```python
from build123d import *

# Parameters (mm, degrees)
SKETCH_1_W                  = 69.5
SKETCH_1_H                  = 55
HOLE_WIZARD_1_D             = 135
HOLE_WIZARD_1_DEPTH         = 13
SKETCH_4_R                  = 15
EXTRUDE_1_DEPTH             = 8
HOLE_WIZARD_M22_1_D         = 26
HOLE_WIZARD_M22_1_DEPTH     = 8
EXTRUDE_2_DEPTH             = 5
CUT_EXTRUDE_START           = -5
CUT_EXTRUDE_1_DEPTH         = 5
CUT_EXTRUDE_2_DEPTH         = 5
CUT_EXTRUDE_3_DEPTH         = 5
HOLE_WIZARD_2_D             = 135
HOLE_WIZARD_2_DEPTH         = 40
THICKEN_START               = -4.2
THICKEN_1_OUTLINE_W         = 3
THICKEN_1_OUTLINE_H         = 6
THICKEN_1_DEPTH             = 8.4
SKETCH_13_W                 = 5
SKETCH_13_H                 = 5
SKETCH_14_W                 = 5
SKETCH_14_H                 = 5
SKETCH_15_W                 = 5
SKETCH_15_H                 = 5
SKETCH_16_W                 = 5
SKETCH_16_H                 = 5
SKETCH_17_W                 = 5
SKETCH_17_H                 = 5
SKETCH_18_W                 = 5
SKETCH_18_H                 = 5
SKETCH_19_W                 = 2.5
SKETCH_19_H                 = 37
SKETCH_20_W                 = 2.5
SKETCH_20_H                 = 37
SKETCH_21_W                 = 2.5
SKETCH_21_H                 = 37
SKETCH_22_W                 = 2.5
SKETCH_22_H                 = 37
HOLE_WIZARD_6_5_6_5_1_D     = 6.5
HOLE_WIZARD_6_5_6_5_1_DEPTH = 3.4
HOLE_WIZARD_15_0_15_1_D     = 15
HOLE_WIZARD_15_0_15_1_DEPTH = 15
HOLE_WIZARD_6_0_6_1_D       = 6
HOLE_WIZARD_6_0_6_1_DEPTH   = 29.048717705
RIB_START                   = -1
RIB_1_OUTLINE_W             = 1
RIB_1_OUTLINE_H             = 4
RIB_1_DEPTH                 = 2
RIB_2_OUTLINE_W             = 4
RIB_2_OUTLINE_H             = 1
RIB_2_DEPTH                 = 2
RIB_3_OUTLINE_W             = 4
RIB_3_OUTLINE_H             = 1
RIB_3_DEPTH                 = 2
RIB_4_OUTLINE_W             = 4
RIB_4_OUTLINE_H             = 1
RIB_4_DEPTH                 = 2


# Read off the part's stored shape, not the designer's step: 切除-加厚1, 筋1, 筋2, 筋3, 筋4
with BuildPart() as part:
    # 草图1 → 旋转1 (revolve)
    with BuildSketch(Plane.XZ, mode=Mode.PRIVATE) as revolve_1_sk:
        with Locations((34.75, 27.5)):
            Rectangle(SKETCH_1_W, SKETCH_1_H)
    revolve(revolve_1_sk.sketch.rotate(Axis((0, 0, 55), (0, 0, -1)), 180), axis=Axis((0, 0, 55), (0, 0, -1)))

    # 孔1
    with Locations(Plane.XY.offset(55)):
        with Locations((0, 0)):
            Hole(HOLE_WIZARD_1_D / 2, depth=HOLE_WIZARD_1_DEPTH)

    # 草图4 → 凸台-拉伸1 (add)
    with BuildSketch(Plane.XY.offset(42)):
        with Locations(Location((0, 0, 0), (0, 0, 180))):
            Circle(SKETCH_4_R)
    extrude(amount=EXTRUDE_1_DEPTH)

    # M22 间隙孔1
    with Locations(Plane.XY.offset(50)):
        with Locations((0, 0)):
            Hole(HOLE_WIZARD_M22_1_D / 2, depth=HOLE_WIZARD_M22_1_DEPTH)

    # 草图7 → 凸台-拉伸2 (add)
    with BuildSketch(Plane.XY.offset(42)):
        with BuildLine():
            Line((12.961481397, -1), (1, -1))
            Line((1, -1), (1, -12.961481397))
            ThreePointArc((1, -12.961481397), (-9.192388155, 9.192388155), (12.961481397, -1))
        make_face()
    extrude(amount=EXTRUDE_2_DEPTH)

    # 草图8 → 切除-拉伸1 (cut)
    with BuildSketch(Plane.XY.offset(47).offset(CUT_EXTRUDE_START)):
        with BuildLine():
            Line((-1, -12.961481397), (-1, -1))
            Line((-1, -1), (-12.961481397, -1))
            ThreePointArc((-12.961481397, -1), (-9.192388155, -9.192388155), (-1, -12.961481397))
        make_face()
    extrude(amount=CUT_EXTRUDE_1_DEPTH, mode=Mode.SUBTRACT)

    # 草图9 → 切除-拉伸2 (cut)
    with BuildSketch(Plane.XY.offset(47).offset(CUT_EXTRUDE_START)):
        with BuildLine():
            Line((-12.961481397, 1), (-1, 1))
            Line((-1, 1), (-1, 12.961481397))
            ThreePointArc((-1, 12.961481397), (-9.192388155, 9.192388155), (-12.961481397, 1))
        make_face()
    extrude(amount=CUT_EXTRUDE_2_DEPTH, mode=Mode.SUBTRACT)

    # 草图10 → 切除-拉伸3 (cut)
    with BuildSketch(Plane.XY.offset(47).offset(CUT_EXTRUDE_START)):
        with BuildLine():
            Line((1, 12.961481397), (1, 1))
            Line((1, 1), (12.961481397, 1))
            ThreePointArc((12.961481397, 1), (9.192388155, 9.192388155), (1, 12.961481397))
        make_face()
    extrude(amount=CUT_EXTRUDE_3_DEPTH, mode=Mode.SUBTRACT)

    # 孔2
    with Locations(Plane(origin=(0, 0, 0), x_dir=(-1, 0, 0), z_dir=(0, 0, -1))):
        with Locations((0, 0)):
            Hole(HOLE_WIZARD_2_D / 2, depth=HOLE_WIZARD_2_DEPTH)

    # 切除-加厚1 outline → 切除-加厚1 (cut)
    with BuildSketch(Plane(origin=(0, 0, 0), x_dir=(0.5591929034707426, 0.8290375725550445, 0), z_dir=(0.8290375725550445, -0.5591929034707428, 0)).offset(THICKEN_START)):
        with Locations((-68.5, 3)):
            Rectangle(THICKEN_1_OUTLINE_W, THICKEN_1_OUTLINE_H)
    extrude(amount=THICKEN_1_DEPTH, mode=Mode.SUBTRACT)

    # 草图13 → 旋转2 (revolve)
    with BuildSketch(Plane.XZ.offset(25), mode=Mode.PRIVATE) as revolve_2_sk:
        with Locations((45.801270189, 44.5)):
            Rectangle(SKETCH_13_W, SKETCH_13_H)
    revolve(revolve_2_sk.sketch.rotate(Axis((43.301270189, -25, 47), (0, 0, -1)), 180), axis=Axis((43.301270189, -25, 47), (0, 0, -1)))

    # 草图14 → 旋转3 (revolve)
    with BuildSketch(Plane.XZ.offset(-25), mode=Mode.PRIVATE) as revolve_3_sk:
        with Locations((45.801270189, 44.5)):
            Rectangle(SKETCH_14_W, SKETCH_14_H)
    revolve(revolve_3_sk.sketch.rotate(Axis((43.301270189, 25, 47), (0, 0, -1)), 180), axis=Axis((43.301270189, 25, 47), (0, 0, -1)))

    # 草图15 → 旋转4 (revolve)
    with BuildSketch(Plane.XZ.offset(-50), mode=Mode.PRIVATE) as revolve_4_sk:
        with Locations((2.5, 44.5)):
            Rectangle(SKETCH_15_W, SKETCH_15_H)
    revolve(revolve_4_sk.sketch.rotate(Axis((0, 50, 47), (0, 0, -1)), 180), axis=Axis((0, 50, 47), (0, 0, -1)))

    # 草图16 → 旋转5 (revolve)
    with BuildSketch(Plane.XZ.offset(-25), mode=Mode.PRIVATE) as revolve_5_sk:
        with Locations((-40.801270189, 44.5)):
            Rectangle(SKETCH_16_W, SKETCH_16_H)
    revolve(revolve_5_sk.sketch.rotate(Axis((-43.301270189, 25, 47), (0, 0, -1)), 180), axis=Axis((-43.301270189, 25, 47), (0, 0, -1)))

    # 草图17 → 旋转6 (revolve)
    with BuildSketch(Plane.XZ.offset(25), mode=Mode.PRIVATE) as revolve_6_sk:
        with Locations((-40.801270189, 44.5)):
            Rectangle(SKETCH_17_W, SKETCH_17_H)
    revolve(revolve_6_sk.sketch.rotate(Axis((-43.301270189, -25, 47), (0, 0, -1)), 180), axis=Axis((-43.301270189, -25, 47), (0, 0, -1)))

    # 草图18 → 旋转7 (revolve)
    with BuildSketch(Plane.XZ.offset(50), mode=Mode.PRIVATE) as revolve_7_sk:
        with Locations((2.5, 44.5)):
            Rectangle(SKETCH_18_W, SKETCH_18_H)
    revolve(revolve_7_sk.sketch.rotate(Axis((0, -50, 47), (0, 0, -1)), 180), axis=Axis((0, -50, 47), (0, 0, -1)))

    # 草图19 → 旋转8 (revolve)
    with BuildSketch(Plane(origin=(0, -11.468398436, 0), x_dir=(1, 0, 0), z_dir=(0, 1, 0))):
        with Locations((-57.749795231, -21.5)):
            Rectangle(SKETCH_19_W, SKETCH_19_H)
    revolve(axis=Axis((-58.999795231, -11.468398436, 3), (0, 0, 1)))

    # 草图20 → 旋转9 (revolve)
    with BuildSketch(Plane(origin=(0, -58.999795231, 0), x_dir=(1, 0, 0), z_dir=(0, 1, 0))):
        with Locations((12.718398436, -21.5)):
            Rectangle(SKETCH_20_W, SKETCH_20_H)
    revolve(axis=Axis((11.468398436, -58.999795231, 3), (0, 0, 1)))

    # 草图21 → 旋转10 (revolve)
    with BuildSketch(Plane(origin=(0, 58.999795231, 0), x_dir=(1, 0, 0), z_dir=(0, 1, 0))):
        with Locations((-10.218398436, -21.5)):
            Rectangle(SKETCH_21_W, SKETCH_21_H)
    revolve(axis=Axis((-11.468398436, 58.999795231, 3), (0, 0, 1)))

    # 草图22 → 旋转11 (revolve)
    with BuildSketch(Plane(origin=(0, 11.468398436, 0), x_dir=(1, 0, 0), z_dir=(0, 1, 0))):
        with Locations((60.249795231, -21.5)):
            Rectangle(SKETCH_22_W, SKETCH_22_H)
    revolve(axis=Axis((58.999795231, 11.468398436, 3), (0, 0, 1)))

    # Ø6.5 (6.5) 直径孔1
    with Locations(Plane.XY.offset(47)):
        with Locations((0, -50), (-43.301270189, -25), (-43.301270189, 25), (0, 50), (43.301270189, 25), (43.301270189, -25)):
            Hole(HOLE_WIZARD_6_5_6_5_1_D / 2, depth=HOLE_WIZARD_6_5_6_5_1_DEPTH)

    # Ø15.0 (15) 直径孔1
    with Locations(Plane(origin=(0, 0, 40), x_dir=(-1, 0, 0), z_dir=(0, 0, -1))):
        with Locations((-30.5, 0)):
            Hole(HOLE_WIZARD_15_0_15_1_D / 2, depth=HOLE_WIZARD_15_0_15_1_DEPTH)

    # Ø6.0 (6) 直径孔1
    with Locations(Plane(origin=(-37.70822303, -55.904739656, 0), x_dir=(0.8290375725550408, -0.5591929034707481, 0), z_dir=(0.5591929034707481, 0.8290375725550408, 0))):
        with Locations((0, -6)):
            Hole(HOLE_WIZARD_6_0_6_1_D / 2, depth=HOLE_WIZARD_6_0_6_1_DEPTH)

    # 筋1 outline → 筋1 (add)
    with BuildSketch(Plane(origin=(0, 0, 0), x_dir=(0, 0, -1), z_dir=(1, 0, 0)).offset(RIB_START)):
        with Locations((-42.5, -16)):
            Rectangle(RIB_1_OUTLINE_W, RIB_1_OUTLINE_H)
    extrude(amount=RIB_1_DEPTH)

    # 筋2 outline → 筋2 (add)
    with BuildSketch(Plane(origin=(0, 0, 0), x_dir=(0, -1, 0), z_dir=(-1, 0, 0)).offset(RIB_START)):
        with Locations((-16, 42.5)):
            Rectangle(RIB_2_OUTLINE_W, RIB_2_OUTLINE_H)
    extrude(amount=RIB_2_DEPTH)

    # 筋3 outline → 筋3 (add)
    with BuildSketch(Plane(origin=(0, 0, 0), x_dir=(1, 0, 0), z_dir=(0, 1, 0)).offset(RIB_START)):
        with Locations((16, -42.5)):
            Rectangle(RIB_3_OUTLINE_W, RIB_3_OUTLINE_H)
    extrude(amount=RIB_3_DEPTH)

    # 筋4 outline → 筋4 (add)
    with BuildSketch(Plane(origin=(0, 0, 0), x_dir=(1, 0, 0), z_dir=(0, 1, 0)).offset(RIB_START)):
        with Locations((-16, -42.5)):
            Rectangle(RIB_4_OUTLINE_W, RIB_4_OUTLINE_H)
    extrude(amount=RIB_4_DEPTH)


solid = part.part
```
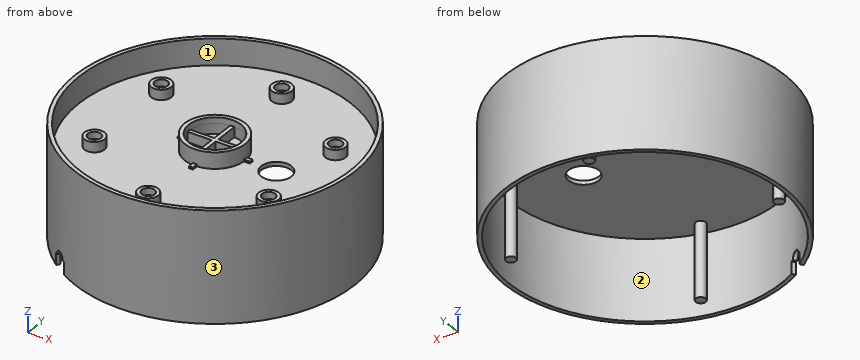
Can you work these out from the model? Positions are in its coordinate system, mm. Face numbers are marked on the shaded views. A direction names the side the tool comes from. Give positions to 0.01 mm unless a question says otherwise; leave off trailing zeros. Order: outer loops, then holes, each group sorted by start corner. A loop starts at its lowest first (then second) coordinate and runs counter-clockwise, first axis right, second up. Notation, with made-up numbers: (29.5, 31.25) - (55.5, 31.25) arc R35 ccw to (55.5, 65.25) - close; hole circle Ø8 at (48, 2). An arc over 180 degrees is marked (long way). Use a Markdown table: item, result. Add a question column.
Q1. I'm going to push flat-ended pins straight in: pin 1 (6 mm diameter, centred on y = 6.5, z = 35.5, fed in from +X); pin 2 (5 mm diameter, centred on x = -43.5, y = 44.5, fed in from +Z); pin 3 (1.5 mm diameter, centred on x = -10.5, y = 51, fed in from -Z). Where does each tip first touch, or does it pass through?
Q2. If we section it at A-A on x = 26: Write out the boundary of the cut face in (y, z), plus the area to 3 significant figures.
Q3. On a 3-axis mill with a long thin cutter (end or side, diameter ignored), from which of +Z, -Z, +X, -X, +Y, -Y can I reach the whole of each face in a straight line? I mean the marked faces 1, 2 and 3. Say none if no direction works.
Q4. If we section it at C-C on y = -50: Write out the boundary of the cut face in (x, z), plus the area to 3 significant figures.
Q5. If we section it at D-D on y = -25: Write out the boundary of the cut face in (x, z).
Q6. Please list where these lines run through material, in increasing order: line 1 along Y through (x, z) = (0, 48); line 2 along Y through (x, z) = (2, 53); line 3 along Y through (x, z) = (-12.5, 35).
Q7. If we section it at B-B on z = 20: Write out the boundary of the cut face in (x, y), plus the area to 3 significant figures.
Answers follow:
| question | item | result |
|---|---|---|
| 1 | pin 1 | stops at x = 69.41 |
| 1 | pin 2 | stops at z = 42 |
| 1 | pin 3 | stops at z = 40 |
| 2 | outline | (-64.45, 0) - (-62.29, 0) - (-62.29, 40) - (-6, 40) - (-6, 42) - (-62.29, 42) - (-62.29, 55) - (-64.45, 55) - close; (6, 40) - (62.29, 40) - (62.29, 0) - (64.45, 0) - (64.45, 55) - (62.29, 55) - (62.29, 42) - (6, 42) - close |
| 2 | area | 463 mm^2 |
| 3 | face 1 | +Z |
| 3 | face 2 | -Z |
| 3 | face 3 | +Z, -Z |
| 4 | outline | (-48.27, 0) - (-45.35, 0) - (-45.35, 40) - (45.35, 40) - (45.35, 0) - (48.27, 0) - (48.27, 55) - (45.35, 55) - (45.35, 42) - (5, 42) - (5, 47) - (3.25, 47) - (3.25, 43.6) - (-3.25, 43.6) - (-3.25, 47) - (-5, 47) - (-5, 42) - (-45.35, 42) - (-45.35, 55) - (-48.27, 55) - close |
| 4 | area | 531 mm^2 |
| 5 | outline | (-64.85, 0) - (-62.7, 0) - (-62.7, 40) - (62.7, 40) - (62.7, 0) - (64.85, 0) - (64.85, 55) - (62.7, 55) - (62.7, 42) - (48.3, 42) - (48.3, 47) - (46.55, 47) - (46.55, 43.6) - (40.05, 43.6) - (40.05, 47) - (38.3, 47) - (38.3, 42) - (-38.3, 42) - (-38.3, 47) - (-40.05, 47) - (-40.05, 43.6) - (-46.55, 43.6) - (-46.55, 47) - (-48.3, 47) - (-48.3, 42) - (-62.7, 42) - (-62.7, 55) - (-64.85, 55) - close |
| 6 | line 1 | y = -69.5 to -67.5, -15 to -13, 13 to 15, 67.5 to 69.5 |
| 6 | line 2 | y = -69.47 to -67.47, 67.47 to 69.47 |
| 6 | line 3 | y = -68.37 to -66.33, 56.72 to 61.28, 66.33 to 68.37 |
| 7 | outline | circle Ø139 at (0, 0); circle Ø5 at (-59, -11.47); circle Ø5 at (-11.47, 59); circle Ø5 at (11.47, -59); circle Ø5 at (59, 11.47); hole circle Ø135 at (0, 0) |
| 7 | area | 939 mm^2 |
